```python
from build123d import *

# Parameters (mm, degrees)
IZIM1_W                          = 60
IZIM1_H                          = 60
Y_KSEKLIK_EKSTR_ZYON1_DEPTH      = 50
IZIM2_R                          = 10
Y_KSEKLIK_EKSTR_ZYON2_DEPTH      = 50
IZIM3_R                          = 4.482666428
Y_KSEKLIK_EKSTR_ZYON3_DEPTH      = 35
Y_KSEKLIK_EKSTR_ZYON4_DEPTH      = 15
PAH1_SIZE                        = 2
Y_KSEKLIK_EKSTR_ZYON7_DEPTH      = 100
Y_KSEKLIK_EKSTR_ZYON7_DEPTH_BACK = 53
IZIM8_R                          = 5
IZIM9_W                          = 60
IZIM9_H                          = 56.52547631
Y_KSEKLIK_EKSTR_ZYON8_DEPTH      = 15
RADYUS2_R                        = 10
Y_KSEKLIK_EKSTR_ZYON9_DEPTH      = 15
Y_KSEKLIK_EKSTR_ZYON9_DEPTH_BACK = 15
IZIM11_R                         = 6.953917593
KES_EKSTR_ZYON1_DEPTH            = 75
RADYUS3_R                        = 5
IZIM12_W                         = 45
IZIM12_H                         = 50
Y_KSEKLIK_EKSTR_ZYON10_DEPTH     = 5
IZIM13_W                         = 45
IZIM13_H                         = 50
Y_KSEKLIK_EKSTR_ZYON11_DEPTH     = 5
IZIM14_R                         = 5
KES_EKSTR_ZYON2_DEPTH            = 98
RADYUS4_R                        = 2


with BuildPart() as part:
    # Çizim1 → Yükseklik-Ekstrüzyon1 (new body)
    with BuildSketch(Plane.XY):
        Rectangle(IZIM1_W, IZIM1_H)
    extrude(amount=Y_KSEKLIK_EKSTR_ZYON1_DEPTH)

    # Çizim2 → Yükseklik-Ekstrüzyon2 (add)
    with BuildSketch(Plane(origin=(0, 0, 0), x_dir=(-1, 0, 0), z_dir=(0, 0, -1))):
        Circle(IZIM2_R)
    extrude(amount=Y_KSEKLIK_EKSTR_ZYON2_DEPTH)

    # Çizim3 → Yükseklik-Ekstrüzyon3 (add)
    with BuildSketch(Plane(origin=(0, 0, -50), x_dir=(-1, 0, 0), z_dir=(0, 0, -1))):
        Circle(IZIM3_R)
    extrude(amount=Y_KSEKLIK_EKSTR_ZYON3_DEPTH)

    # Çizim4 → Yükseklik-Ekstrüzyon4 (add)
    with BuildSketch(Plane(origin=(0, 0, -85), x_dir=(-1, 0, 0), z_dir=(0, 0, -1))):
        Polygon((9.810169594, -1.939219571), (6.584498209, 7.526246298), (-3.225671385, 9.465465869), (-9.810169594, 1.939219571), (-6.584498209, -7.526246298), (3.225671385, -9.465465869), align=None)
    extrude(amount=Y_KSEKLIK_EKSTR_ZYON4_DEPTH)

    # Pah1
    pah1_edges = [part.edges().sort_by_distance(p)[0] for p in [
        (-6.517920489, -5.70234272, -100),
        (-8.197333901, 2.793513364, -100),
        (-1.679413412, 8.495856084, -100),
        (6.517920489, 5.70234272, -100),
        (8.197333901, -2.793513364, -100),
        (1.679413412, -8.495856084, -100),
    ]]
    chamfer(pah1_edges, length=PAH1_SIZE)

    # Çizim8 → Yükseklik-Ekstrüzyon7 (add, two sides: drawn at the far end of the back side and taken through both)
    with BuildSketch(Plane(origin=(0, 0, 0), x_dir=(-1, 0, 0), z_dir=(0, 0, -1)).offset(-Y_KSEKLIK_EKSTR_ZYON7_DEPTH_BACK)):
        with Locations((-22.5, 22.5)):
            Circle(IZIM8_R)
        with Locations((22.5, 22.5)):
            Circle(IZIM8_R)
        with Locations((22.5, -22.5)):
            Circle(IZIM8_R)
        with Locations((-22.5, -22.5)):
            Circle(IZIM8_R)
    extrude(amount=Y_KSEKLIK_EKSTR_ZYON7_DEPTH + Y_KSEKLIK_EKSTR_ZYON7_DEPTH_BACK)

    # Çizim9 → Yükseklik-Ekstrüzyon8 (add)
    with BuildSketch(Plane(origin=(0, 0, -100), x_dir=(-1, 0, 0), z_dir=(0, 0, -1))):
        Rectangle(IZIM9_W, IZIM9_H)
    extrude(amount=Y_KSEKLIK_EKSTR_ZYON8_DEPTH)

    # Radyus2
    radyus2_edges = [part.edges().sort_by_distance(p)[0] for p in [
        (30, 28.262738155, -107.5),
        (30, -28.262738155, -107.5),
        (-30, -28.262738155, -107.5),
        (-30, 28.262738155, -107.5),
    ]]
    fillet(radyus2_edges, radius=RADYUS2_R)

    # Çizim10 → Yükseklik-Ekstrüzyon9 (add, two sides: drawn at the far end of the back side and taken through both)
    with BuildSketch(Plane(origin=(0, 0, 0), x_dir=(1, 0, 0), z_dir=(0, 1, 0)).offset(-Y_KSEKLIK_EKSTR_ZYON9_DEPTH_BACK)):
        Polygon((30, -50), (30, -90), (-30, -50), align=None)
    extrude(amount=Y_KSEKLIK_EKSTR_ZYON9_DEPTH + Y_KSEKLIK_EKSTR_ZYON9_DEPTH_BACK)

    # Çizim11 → Kes-Ekstrüzyon1 (cut)
    with BuildSketch(Plane(origin=(30, 0, 0), x_dir=(0, 0, -1), z_dir=(1, 0, 0))):
        with Locations(Location((-68.644638819, 0, 0), (0, 0, 90))):
            Circle(IZIM11_R)
    extrude(amount=-KES_EKSTR_ZYON1_DEPTH, mode=Mode.SUBTRACT)

    # Radyus3
    radyus3_edges = [part.edges().sort_by_distance(p)[0] for p in [
        (-30, 30, 25),
        (30, 30, 25),
        (30, -30, 25),
        (-30, -30, 25),
    ]]
    fillet(radyus3_edges, radius=RADYUS3_R)

    # Çizim12 → Yükseklik-Ekstrüzyon10 (add)
    with BuildSketch(Plane.XZ.offset(30)):
        with Locations((47.5, 25)):
            Rectangle(IZIM12_W, IZIM12_H)
    extrude(amount=-Y_KSEKLIK_EKSTR_ZYON10_DEPTH)

    # Çizim13 → Yükseklik-Ekstrüzyon11 (add)
    with BuildSketch(Plane(origin=(0, 30, 0), x_dir=(1, 0, 0), z_dir=(0, 1, 0))):
        with Locations((47.5, -25)):
            Rectangle(IZIM13_W, IZIM13_H)
    extrude(amount=-Y_KSEKLIK_EKSTR_ZYON11_DEPTH)

    # Çizim14 → Kes-Ekstrüzyon2 (cut)
    with BuildSketch(Plane(origin=(0, 30, 0), x_dir=(1, 0, 0), z_dir=(0, 1, 0))):
        with Locations(Location((50, -12.123765205, 0), (0, 0, 180))):
            Circle(IZIM14_R)
        with Locations(Location((50, -36.123765205, 0), (0, 0, 180))):
            Circle(IZIM14_R)
    extrude(amount=-KES_EKSTR_ZYON2_DEPTH, mode=Mode.SUBTRACT)

    # Radyus4
    # the kernel refuses this fillet: 2 mm, written as the material it adds along each edge
    with BuildSketch(Plane(origin=(-30, -15, 50), x_dir=(0, -1, 0), z_dir=(1, 0, 0))) as radyus4_piece_1_section:
        with BuildLine():
            CenterArc((RADYUS4_R, -RADYUS4_R), RADYUS4_R, 90, 90)
            Line((0, -RADYUS4_R), (0, 0))
            Line((0, 0), (RADYUS4_R, 0))
        make_face()
    radyus4_piece_1 = extrude(amount=60, mode=Mode.PRIVATE)
    radyus4_piece_1 = split(radyus4_piece_1, bisect_by=Plane(origin=(-8.790437834, -15.455546118, 64.139708111), z_dir=(0.5547001962252291, 0, -0.8320502943378437)), keep=Keep.TOP, mode=Mode.PRIVATE)
    add(radyus4_piece_1)
    with BuildSketch(Plane(origin=(-30, 15, 50), x_dir=(0, 1, 0), z_dir=(1, 0, 0))) as radyus4_piece_2_section:
        with BuildLine():
            CenterArc((RADYUS4_R, RADYUS4_R), RADYUS4_R, 180, 90)
            Line((0, RADYUS4_R), (0, 0))
            Line((0, 0), (RADYUS4_R, 0))
        make_face()
    radyus4_piece_2 = extrude(amount=60, mode=Mode.PRIVATE)
    radyus4_piece_2 = split(radyus4_piece_2, bisect_by=Plane(origin=(-8.790437834, 15.455546118, 64.139708111), z_dir=(0.5547001962252291, 0, -0.8320502943378437)), keep=Keep.TOP, mode=Mode.PRIVATE)
    add(radyus4_piece_2)


solid = part.part
```
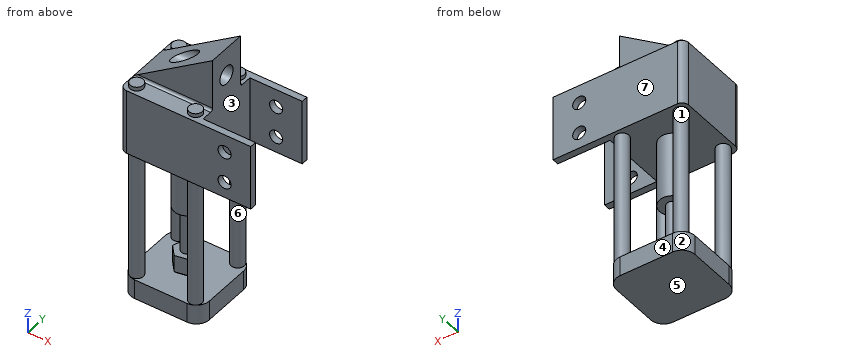
Verification items for the finished model (mm, model axes). Face numbers are marked on the shaded views. A direction names the side the tool comes from. Give positions to 0.01 mm unless a question says otherwise; leave off trailing zeros. Order: outer loops, then holes, each group sorted by start corner. A loop starts at its lowest first (then second) coordinate and runs counter-clockwise, first axis right, second up. Notation, with made-up numbers: M 19.25,-37.5 L 68.25,-37.5 A26 cw 68.25,1.5 Z; hole C -19.75,-17.5 d11. An arc over 180 degrees is marked long. Return JSON: item names as keys, results as strings. Group by question number.
1) Section check D-D on z = 43.5. Record the cut outline in (x, y).
2) Section check A-A on x = 32. Record the cut outline in (y, z).
3) Section check C-C on x = 50. Record the cut outline in (y, z), and give its area (3 significant figures).
4) Access from +Z, -Z, +X, -X, +Y, -Y to the whole of each face (thin tool, end or side, straight path). Record for the marked faces 1, 2, 3 and 4.
5) Mould release check, pull along Z, two halves, no side actions. Record for the marked faces 5, 6 and 7: pulls with the +Z half, pulls with the -Z half, needs draft (parallel to the pull), parting line crosses it, or undercut.
6) Section check B-B on z = -7.5. Record the cut outline in (x, y).
7) Scan lines: line 1 (Z direction, x = 50, y = -27); line 2 (Y direction, x = -22.5, z = -71.5); line 3 (Y direction, x = 54, z = 28). Record each from-to range of solid material in increasing order.
8) Go/stop test with flat-tipped pins: pin 1 Ø4.5 at (y, z) = (8.5, -108.5) entering from +X; pin 2 Ø8 at (x, y) = (27.5, 22) entering from +Z; pin 3 Ø5 at (x, z) = (25, 66.5) entering from +Y; pin 4 Ø16 at (x, z) = (50, 12.12) entering from +Y. Record where each tip stops, or that it passes through.
Answer block:
{
 "1": {"outline": "M -30,-25 A5 ccw -25,-30 L 70,-30 L 70,-25 L 30,-25 L 30,25 L 70,25 L 70,30 L -25,30 A5 ccw -30,25 Z"},
 "2": {"outline": "M -30,0 L -25,0 L -25,50 L -30,50 Z; M 25,0 L 30,0 L 30,50 L 25,50 Z"},
 "3": {"outline": "M -30,0 L -25,0 L -25,7.12 L -30,7.12 Z; M -30,17.12 L -25,17.12 L -25,31.12 L -30,31.12 Z; M -30,41.12 L -25,41.12 L -25,50 L -30,50 Z; M 25,0 L 30,0 L 30,7.12 L 25,7.12 Z; M 25,17.12 L 30,17.12 L 30,31.12 L 25,31.12 Z; M 25,41.12 L 30,41.12 L 30,50 L 25,50 Z", "area": "300 mm^2"},
 "4": {"face 1": "none", "face 2": "-Z, -X, +Y", "face 3": "+Z, -Z, +X", "face 4": "-Z, +X, -X, +Y"},
 "5": {"face 5": "pulls with the -Z half", "face 6": "undercut", "face 7": "needs draft"},
 "6": {"outline": "C -22.5,-22.5 d10; C -22.5,22.5 d10; C 0,0 d20; C 22.5,-22.5 d10; C 22.5,22.5 d10"},
 "7": {"line 1": "z = 0 to 7.12, 17.12 to 31.12, 41.12 to 50", "line 2": "y = -27.5 to -17.5, 17.5 to 27.5", "line 3": "y = -30 to -25, 25 to 30"},
 "8": {"pin 1": "stops at x = 30", "pin 2": "stops at z = 53", "pin 3": "stops at y = 15", "pin 4": "stops at y = 30"}
}
